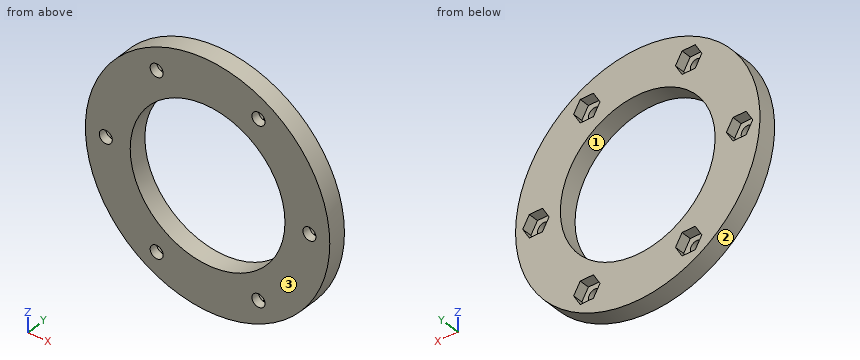
```python
from build123d import *

# Parameters (mm, degrees)
SKETCH1_R           = 30
SKETCH1_R_2         = 19
SKETCH1_R_3         = 1.6
BOSS_EXTRUDE1_DEPTH = 2
SKETCH2_R           = 30
SKETCH2_R_2         = 19
BOSS_EXTRUDE3_DEPTH = 2.5


with BuildPart() as part:
    # Sketch1 → Boss-Extrude1 (new body)
    with BuildSketch(Plane(origin=(0, 0, 0), x_dir=(1, 0, 0), z_dir=(0, 1, 0))):
        Circle(SKETCH1_R)
        Circle(SKETCH1_R_2, mode=Mode.SUBTRACT)
        with Locations((25, 0)):
            Circle(SKETCH1_R_3, mode=Mode.SUBTRACT)
        with Locations((12.5, -21.650635095)):
            Circle(SKETCH1_R_3, mode=Mode.SUBTRACT)
        with Locations((-12.5, -21.650635095)):
            Circle(SKETCH1_R_3, mode=Mode.SUBTRACT)
        with Locations((-25, 0)):
            Circle(SKETCH1_R_3, mode=Mode.SUBTRACT)
        with Locations((-12.5, 21.650635095)):
            Circle(SKETCH1_R_3, mode=Mode.SUBTRACT)
        with Locations((12.5, 21.650635095)):
            Circle(SKETCH1_R_3, mode=Mode.SUBTRACT)
    extrude(amount=BOSS_EXTRUDE1_DEPTH)

    # Sketch2 → Boss-Extrude3 (add)
    with BuildSketch(Plane(origin=(0, 2, 0), x_dir=(1, 0, 0), z_dir=(0, 1, 0))):
        Circle(SKETCH2_R)
        Circle(SKETCH2_R_2, mode=Mode.SUBTRACT)
        Polygon((14.116580754, -24.450635095), (15.733161507, -21.650635095), (14.116580754, -18.850635095), (10.883419246, -18.850635095), (9.266838493, -21.650635095), (10.883419246, -24.450635095), align=None, mode=Mode.SUBTRACT)
        Polygon((28.233161507, 0), (26.616580754, 2.8), (23.383419246, 2.8), (21.766838493, 0), (23.383419246, -2.8), (26.616580754, -2.8), align=None, mode=Mode.SUBTRACT)
        Polygon((-14.116580754, -24.450635095), (-10.883419246, -24.450635095), (-9.266838493, -21.650635095), (-10.883419246, -18.850635095), (-14.116580754, -18.850635095), (-15.733161507, -21.650635095), align=None, mode=Mode.SUBTRACT)
        Polygon((-28.233161507, 0), (-26.616580754, -2.8), (-23.383419246, -2.8), (-21.766838493, 0), (-23.383419246, 2.8), (-26.616580754, 2.8), align=None, mode=Mode.SUBTRACT)
        Polygon((-14.116580754, 24.450635095), (-15.733161507, 21.650635095), (-14.116580754, 18.850635095), (-10.883419246, 18.850635095), (-9.266838493, 21.650635095), (-10.883419246, 24.450635095), align=None, mode=Mode.SUBTRACT)
        Polygon((14.116580754, 24.450635095), (10.883419246, 24.450635095), (9.266838493, 21.650635095), (10.883419246, 18.850635095), (14.116580754, 18.850635095), (15.733161507, 21.650635095), align=None, mode=Mode.SUBTRACT)
    extrude(amount=BOSS_EXTRUDE3_DEPTH)


solid = part.part
```
Input: part model. Units: mm. Frame: model coordinates. Face numbers are marked on the shaded views. Coordinates: 2 decimals unless noted, no trailing zeros. Loops run counter-clockwise (first coordinate to the right, second up) from the corner with the lowest first, then second, coordinate; pieces in that order, holes last. Notation, with made-up numbers: M 46.25,26.25 L 102.25,26.25 A14 cw 102.25,46.25 Z; hole C -29.5,26 d10. An arc over 180 degrees is marked long. Answer in a Markdown table with one row per item.
1. Section A-A, the plane y = 0.7. Output: boundary loops of the cut face in (x, z).
Response:
| item | result |
|---|---|
| outline | C 0,0 d60; hole C -25,0 d3.2; hole C 0,0 d38; hole C -12.5,-21.65 d3.2; hole C -12.5,21.65 d3.2; hole C 12.5,-21.65 d3.2; hole C 12.5,21.65 d3.2; hole C 25,0 d3.2 |
2. Material intervals for line 1 (X direction, y = 2.75, z = 0); line 2 (X direction, y = 0.9, z = 0); line 3 (X direction, y = 2.95, z = -22), sorted ascending.
Response:
| item | result |
|---|---|
| line 1 | x = -30 to -28.23, -21.77 to -19, 19 to 21.77, 28.23 to 30 |
| line 2 | x = -30 to -26.6, -23.4 to -19, 19 to 23.4, 26.6 to 30 |
| line 3 | x = -20.4 to -15.53, -9.47 to 9.47, 15.53 to 20.4 |
3. Draft query along X for the marked faces 1, 2 and 3. Return one class per face: pulls with the +X half, pulls with the -X half, needs draft (parallel to the pull), parting line crosses it, or undercut.
Response:
| item | result |
|---|---|
| face 1 | undercut |
| face 2 | parting line crosses it |
| face 3 | needs draft |
4. First-contact query: pin 1 (6 mm diameter, centred on x = 12, z = 23, fed in from +Y); pin 2 (3.5 mm diameter, centred on x = 25, z = 0, fed in from +Y); pin 3 (1 mm diameter, centred on x = 21.5, y = 1.5, fed in from -Z); pin 4 (0.8 mm diameter, centred on x = -13, y = 3.5, fed in from +Z). Flat tips, straight axial feed; report the tip coordinate or a pass-through.
Response:
| item | result |
|---|---|
| pin 1 | stops at y = 4.5 |
| pin 2 | stops at y = 2 |
| pin 3 | stops at z = -21.42 |
| pin 4 | stops at z = 27.23 |
5. Section D-D, the plane x = -12. Output: boundary loops of the cut face in (y, z).
Response:
| item | result |
|---|---|
| outline | M 0,-27.5 L 4.5,-27.5 L 4.5,-24.45 L 2,-24.45 L 2,-23.17 L 0,-23.17 Z; M 0,-20.13 L 2,-20.13 L 2,-18.85 L 4.5,-18.85 L 4.5,-14.73 L 0,-14.73 Z; M 0,14.73 L 4.5,14.73 L 4.5,18.85 L 2,18.85 L 2,20.13 L 0,20.13 Z; M 0,23.17 L 2,23.17 L 2,24.45 L 4.5,24.45 L 4.5,27.5 L 0,27.5 Z |
6. Section C-C, the plane z = -10. Output: boundary loops of the cut face in (x, y), then the cut area to 3 significant figures.
Response:
| item | result |
|---|---|
| outline | M -28.28,0 L -16.16,0 L -16.16,4.5 L -28.28,4.5 Z; M 16.16,0 L 28.28,0 L 28.28,4.5 L 16.16,4.5 Z |
| area | 109 mm2 |
7. Section B-B, the plane x = 0. Output: boundary loops of the cut face in (y, z).
Response:
| item | result |
|---|---|
| outline | M 0,-30 L 4.5,-30 L 4.5,-19 L 0,-19 Z; M 0,19 L 4.5,19 L 4.5,30 L 0,30 Z |
